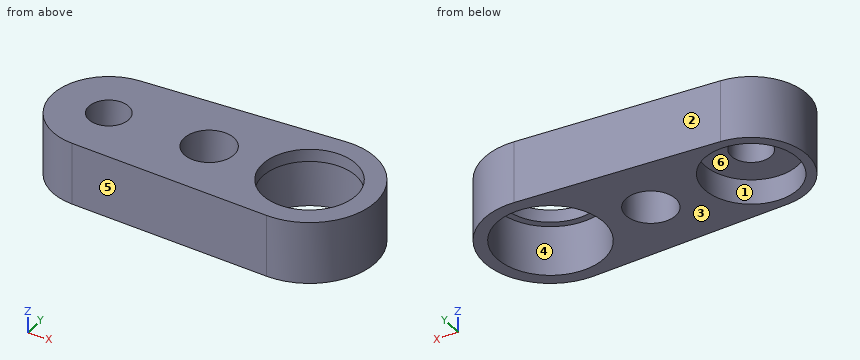
```python
from build123d import *

# Parameters (mm, degrees)
SKETCH_R        = 3.2
SKETCH_R_2      = 7.5
SKETCH_R_3      = 4
PAD_DEPTH       = 10
SKETCH001_R     = 8.6
POCKET_DEPTH    = 8
SKETCH002_R     = 7.5
POCKET001_DEPTH = 4


with BuildPart() as part:
    # Sketch → Pad (new body)
    with BuildSketch(Plane.XY):
        with BuildLine():
            ThreePointArc((-32.45, 8.988743), (-41, 0), (-32.45, -8.988743))
            Line((-32.45, -8.988743), (-0.53, -10.586742))
            ThreePointArc((-0.53, -10.586742), (10.6, 0), (-0.53, 10.586742))
            Line((-32.45, 8.988743), (-0.53, 10.586742))
        make_face()
        with Locations((-32, 0)):
            Circle(SKETCH_R, mode=Mode.SUBTRACT)
        Circle(SKETCH_R_2, mode=Mode.SUBTRACT)
        with Locations((-16, 0)):
            Circle(SKETCH_R_3, mode=Mode.SUBTRACT)
    extrude(amount=PAD_DEPTH)

    # Sketch001 → Pocket (cut)
    with BuildSketch(Plane(origin=(0, 0, 0), x_dir=(1, 0, 0), z_dir=(0, 0, -1))):
        Circle(SKETCH001_R)
    extrude(amount=-POCKET_DEPTH, mode=Mode.SUBTRACT)

    # Sketch002 → Pocket001 (cut)
    with BuildSketch(Plane(origin=(0, 0, 0), x_dir=(1, 0, 0), z_dir=(0, 0, -1))):
        with Locations((-32, 0)):
            Circle(SKETCH002_R)
    extrude(amount=-POCKET001_DEPTH, mode=Mode.SUBTRACT)


solid = part.part
```
Geometry: final body of the model. Coordinates: model frame, mm. Face numbers are marked on the shaded views. A direction names the side the tool comes from. Coordinates: 2 decimals unless noted, no trailing zeros. Order: outer loops, then holes, each group sorted by start corner. A loop starts at its lowest first (then second) coordinate and runs counter-clockwise, first axis right, second up.
Item 1: Section query C-C (z = 7). Output: boundary loops of the cut face in (x, y), then the cut area to 3 significant figures.
Answer:
outline: (-32.45, -8.99) - (-0.53, -10.59) arc R10.6 ccw (long way) to (-0.53, 10.59) - (-32.45, 8.99) arc R9 ccw to start; hole circle Ø6.4 at (-32, 0); hole circle Ø8 at (-16, 0); hole circle Ø17.2 at (0, 0)
area: 617 mm2
Item 2: Draft query along Y for the marked faces 1, 2, 3 and 4. Return one class per face: released by +Y, released by -Y, zero draft, split by the parting line, or undercut.
Answer:
face 1: undercut
face 2: released by +Y
face 3: zero draft
face 4: undercut
Item 3: Section query B-B (y = 0). Output: boundary loops of the cut face in (x, z).
Answer:
outline: (-41, 0) - (-39.5, 0) - (-39.5, 4) - (-35.2, 4) - (-35.2, 10) - (-41, 10) - close; (-28.8, 4) - (-24.5, 4) - (-24.5, 0) - (-20, 0) - (-20, 10) - (-28.8, 10) - close; (-12, 0) - (-8.6, 0) - (-8.6, 8) - (-7.5, 8) - (-7.5, 10) - (-12, 10) - close; (7.5, 8) - (8.6, 8) - (8.6, 0) - (10.6, 0) - (10.6, 10) - (7.5, 10) - close
Item 4: Section query A-A (x = 0). Output: boundary loops of the cut face in (y, z), then the cut area to 3 significant figures.
Answer:
outline: (-10.6, 0) - (-8.6, 0) - (-8.6, 8) - (-7.5, 8) - (-7.5, 10) - (-10.6, 10) - close; (7.5, 8) - (8.6, 8) - (8.6, 0) - (10.6, 0) - (10.6, 10) - (7.5, 10) - close
area: 44.4 mm2
Item 5: Contact query for flat-ended pins moving along their axis: P1, Ø5, axis at x = -16, y = 0, coming from the +Z side; P2, Ø5, axis at x = -15.5, z = 2, coming from the +Y side; P3, Ø1, axis at x = -10.5, z = 7.5, coming from the -Y side; P4, Ø5, axis at x = -35.5, z = 8.5, coming from the -Y side. Output: stop coordinate, or through.
Answer:
P1: passes through
P2: stops at y = 9.96
P3: stops at y = -10.11
P4: stops at y = -8.94
Item 6: Access query for the marked faces 5 and 6. Directions: +Z, -Z, +X, -X, +Y, -Y. A direction counts if a zero-diameter tool reaches every point of the face in a straight line with its end or side. Return the directions, or none.
Answer:
face 5: +Z, -Z, -X, -Y
face 6: -Z
Item 7: Material intervals for line 1 along X through (y, z) = (2.5, 8.25); line 2 along X through (y, z) = (-0.5, 3.5); line 3 along Y through (x, z) = (-3.5, 4.75), sorted ascending.
Answer:
line 1: x = -40.65 to -34, -30 to -19.12, -12.88 to -7.07, 7.07 to 10.3
line 2: x = -40.99 to -39.48, -24.52 to -19.97, -12.03 to -8.59, 8.59 to 10.59
line 3: y = -10.44 to -7.86, 7.86 to 10.44
Item 8: Section query D-D (y = -7). Output: boundary loops of the cut face in (x, z), then the cut area to 3 significant figures.
Answer:
outline: (-37.66, 0) - (-34.69, 0) - (-34.69, 4) - (-29.31, 4) - (-29.31, 0) - (-5, 0) - (-5, 8) - (-2.69, 8) - (-2.69, 10) - (-37.66, 10) - close; (2.69, 8) - (5, 8) - (5, 0) - (7.96, 0) - (7.96, 10) - (2.69, 10) - close
area: 344 mm2
